Here's the drawing with two shaded views (mm, measured from the low corner). I have some questions. Coordinates: 2 decimals unless noted, no trailing zeros. Loops run counter-clockwise (first coordinate to the right, second up) from the corner with the lowest first, then second, coordinate; pieces in that order, holes last.
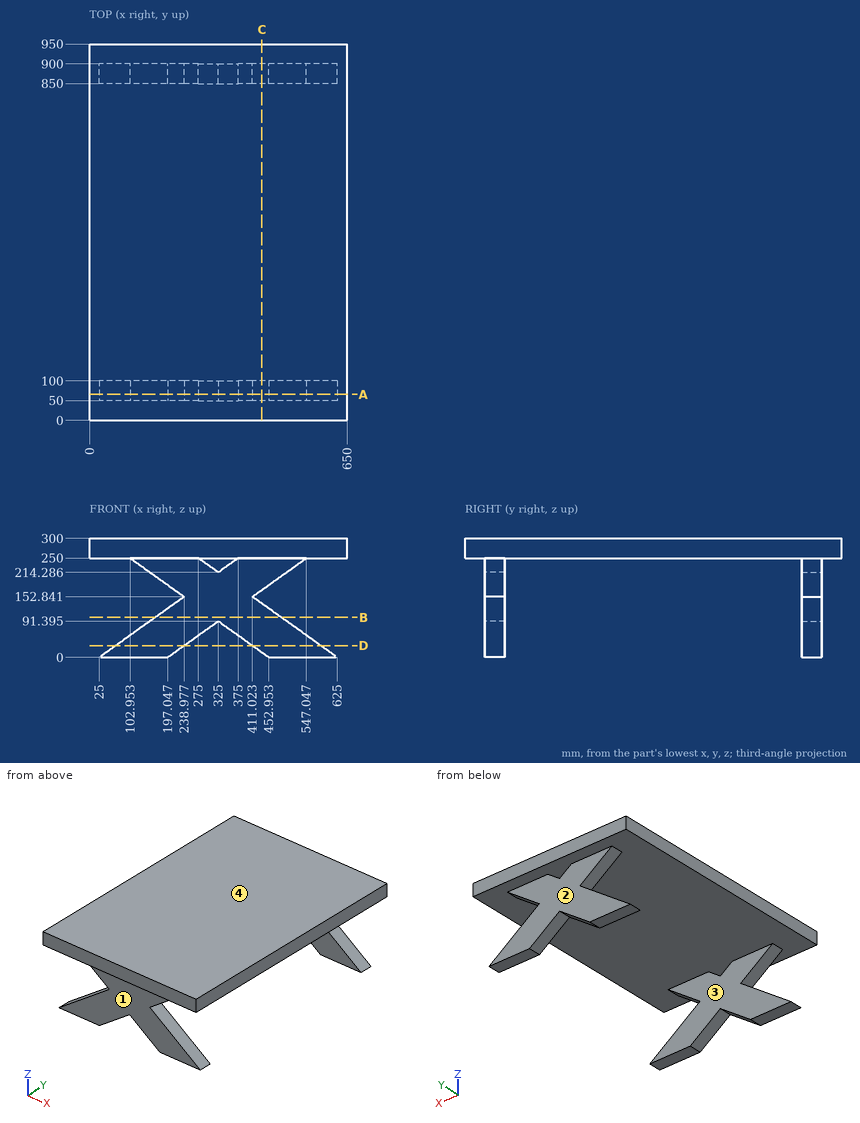
(1) I'm going to push flat-ended pins straight in: pin 1 (3 mm diameter, centred on x = 278, z = 98.5, fed in from +Y); pin 2 (4 mm diameter, centred on x = 78, y = 793, fed in from -Z). Where does each tip first touch, or does it pass through?
Check values:
pin 1: stops at y = 900
pin 2: stops at z = 250
(2) If I drill on probe 1 along Y at (x, z) = (403, 167); probe 2 along Z at (x, y) = (308, 553.5); probe 3 along Z at (x, y) = (381, 55.5) (1 decimal), over which ranges is the centre line in solid material (lowest first)?
Check values:
probe 1: y = 50 to 100, 850 to 900
probe 2: z = 250 to 300
probe 3: z = 51.4 to 300
(3) I want a section at A-A on y = 66. Write out the boundary of the cut face in (x, z) (1 decimal), then the cut area to 3 significant figures.
Check values:
outline: (0, 250) - (103, 250) - (239, 152.8) - (25, 0) - (197, 0) - (325, 91.4) - (453, 0) - (625, 0) - (411, 152.8) - (547, 250) - (650, 250) - (650, 300) - (0, 300) - close; hole (275, 250) - (325, 214.3) - (375, 250) - close
area: 108,000 mm2
(4) I want a section at D-D on z = 29.5. Write out the boundary of the cut face in (x, y), then the cut area to 3 significant figures.
Check values:
outline: (66.3, 50) - (238.35, 50) - (238.35, 100) - (66.3, 100) - close; (66.3, 850) - (238.35, 850) - (238.35, 900) - (66.3, 900) - close; (411.65, 50) - (583.7, 50) - (583.7, 100) - (411.65, 100) - close; (411.65, 850) - (583.7, 850) - (583.7, 900) - (411.65, 900) - close
area: 34,400 mm2
(5) I want a section at B-B on z = 101. Write out the boundary of the cut face in (x, y).
Check values:
outline: (166.4, 50) - (483.6, 50) - (483.6, 100) - (166.4, 100) - close; (166.4, 850) - (483.6, 850) - (483.6, 900) - (166.4, 900) - close
(6) I want a section at C-C on x = 435. Write out the boundary of the cut face in (y, z) (1 decimal), then the cut area to 3 significant figures.
Check values:
outline: (0, 250) - (50, 250) - (50, 170) - (100, 170) - (100, 250) - (850, 250) - (850, 170) - (900, 170) - (900, 250) - (950, 250) - (950, 300) - (0, 300) - close; (50, 12.8) - (100, 12.8) - (100, 135.7) - (50, 135.7) - close; (850, 12.8) - (900, 12.8) - (900, 135.7) - (850, 135.7) - close
area: 67,800 mm2
(7) If we mould it in two halves opening along Y, with no side actions, what happens to the marked faces 1, 2, 3 and 4? For each: released by +Y, released by -Y, zero draft, split by the parting line, or undercut.
Check values:
face 1: released by -Y
face 2: released by +Y
face 3: undercut
face 4: zero draft
